Autodesk Inventor part; units mm, degrees
ref_plane "YZ Plane" through (0, 0, 0) normal (1, 0, 0) x (0, 1, 0)
ref_plane "XZ Plane" through (0, 0, 0) normal (0, 1, 0) x (-1, 0, 0)
ref_plane "XY Plane" through (0, 0, 0) normal (0, 0, 1) x (1, 0, 0)
sketch "Sketch1" plane through (0, 0, 0) normal (1, 0, 0) x (0, 1, 0)
  line L0 (-420.7488, 12.7) -> (420.7488, 12.7) construction
  line L1 (420.7488, 12.7) -> (420.7488, -12.7)
  line L2 (420.7488, -12.7) -> (-420.7488, -12.7) construction
  line L3 (-420.7488, -12.7) -> (-420.7488, 12.7)
  line L4 (0, 0) -> (0, -26.6192) construction
  circle A0 centre (0, -26.6192) radius 3.302
  line L5 (420.7488, 0) -> (-420.7488, 0) construction
  circle A1 centre (38.1, 26.6192) radius 3.302
  circle A2 centre (-76.2, 26.6192) radius 3.302
  line L6 (38.1, 26.6192) -> (-76.2, 26.6192) construction
  line L7 (0, 0) -> (0, 26.6192) construction
  circle A3 centre (0, -26.6192) radius 15.875 construction
  circle A4 centre (38.1, 26.6192) radius 15.875 construction
  circle A5 centre (-76.2, 26.6192) radius 15.875 construction
  line L8 (0, -26.6192) -> (-76.2, 26.6192) construction
  arc A6 (45.8458, 21.0759) -> (38.1, 36.1442) centre (38.1, 26.6192) ccw
  arc A7 (-76.2, 36.1442) -> (-81.6552, 18.8111) centre (-76.2, 26.6192) ccw
  line L9 (38.1, 36.1442) -> (-76.2, 36.1442)
  line L10 (45.8458, 21.0759) -> (7.7458, -32.1625)
  line L11 (-5.4552, -34.4273) -> (-81.6552, 18.8111)
  arc A8 (-5.4552, -34.4273) -> (7.7458, -32.1625) centre (0, -26.6192) ccw
  dimension "d0" = 25.4
  dimension "d1" = 6.604
  dimension "d2" = 13.9192
  dimension "d3" = 31.75
  dimension "d4" = 38.1
  dimension "d5" = 76.2
  dimension "d6" = 9.525
extrude "Extrusion1" add sketch "Sketch1" along normal blind 6.35
properties part number "carriage plate" material "Aluminum 6061"
Verification items for the finished model (mm, model axes). Round coordinates to 2 decimals unless told otherwise and drop trailing zeros. Order: outer loops, then holes, each group sorted by start corner. A loop starts at its lowest first (then second) coordinate and runs counter-clockwise, first axis right, second up.
1. Section check A-A on y = 0. Record the cut outline in (x, z).
Final values:
outline: (0, -36.14) - (6.35, -36.14) - (6.35, -29.92) - (0, -29.92) - close; (0, -23.32) - (6.35, -23.32) - (6.35, 36.14) - (0, 36.14) - close
2. Thickness scan on L1, parallel to Z at x = 4, y = -50; L2, parallel to Z at x = 2.5, y = 37.5; L3, parallel to Z at x = 4.25, y = 38.1. Record the ranges inside material, lowest first.
Final values:
L1: z = -3.31 to 36.14
L2: z = 9.41 to 23.37, 29.87 to 36.14
L3: z = 10.25 to 23.32, 29.92 to 36.14
3. Section check B-B on x = 4. State how many separate pieces and enclosed holes the cut face has, then the cut area to 3 significant figures.
Final values:
separate pieces: 1
enclosed holes: 3
area: 5,820 mm2
4. Section check D-D on y = -71. Record the cut outline in (x, z), then the cut area to 3 significant figures.
Final values:
outline: (0, 11.37) - (6.35, 11.37) - (6.35, 36.14) - (0, 36.14) - close
area: 157 mm2
5. Go/stop test with flat-tipped pins: P1, Ø2, axis at x = 5, z = -23.5, coming from the -Y side; P2, Ø3, axis at y = -51, z = 25.5, coming from the -X side; P3, Ø3, axis at x = 3, y = -27, coming from the -Z side; P4, Ø1, axis at x = 5.5, z = -18.5, coming from the +Y side. Record where each tip stops, or that it passes through.
Final values:
P1: stops at y = -22.53
P2: stops at x = 0
P3: stops at z = -20.42
P4: stops at y = 17.88
6. Section check C-C on z = 4.5. Record the cut outline in (x, y), then the cut area to 3 significant figures.
Final values:
outline: (0, -61.17) - (6.35, -61.17) - (6.35, 33.98) - (0, 33.98) - close
area: 604 mm2
7. Release check for a two-part mould opening along Z. For faces 1 (the flat face through (3.131, 27.062, -5.171)), 2 (the flat face through (3, -18, 36.144)), 3 (the cylindrical face through (3.13, -73.05, 25.63)) record: +Z half, -Z half, draft (parallel to the pull), parting line (faces both ways), or undercut.
Final values:
face 1: -Z half
face 2: +Z half
face 3: undercut
